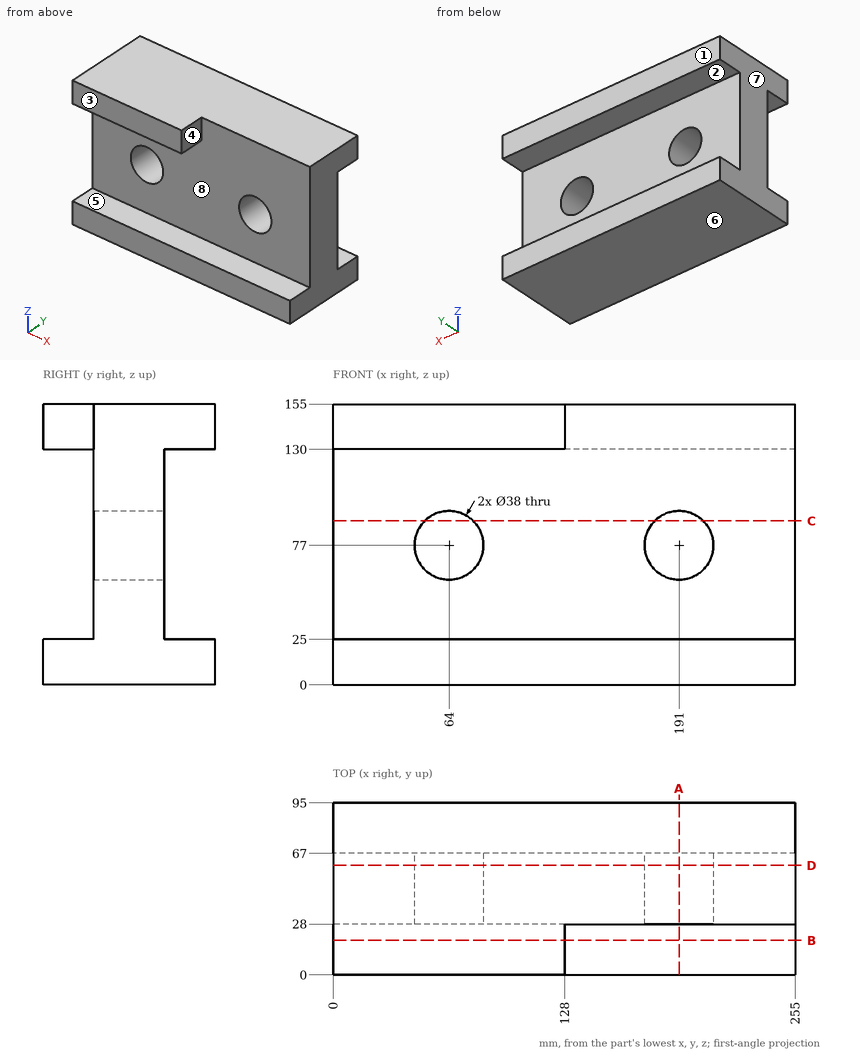
Geometry check sheet. Reference: drawing and pictorial views, mm from the part's lowest x, y, z. A direction names the side the tool comes from. Give positions to 0.01 mm unless a question says otherwise; leave off trailing zeros. Order: outer loops, then holes, each group sorted by start corner. A loop starts at its lowest first (then second) coordinate and runs counter-clockwise, first axis right, second up. Notation, with made-up numbers: M 42.5,55 L 84.5,55 A13 cw 84.5,76 Z; hole C 26,39 d5. An arc over 180 degrees is marked long. Answer as CSV lines item,"result". Start each with the question number.
Item 1: Cross-section at B-B on y = 19. Enter the section's corners in (x, z), plus the area to 4 significant figures.
Item 2: Tool access check on the marked faces 1, 2, 3, 4 and 5. Record the directions out of +Z, -Z, +X, -X, +Y, -Y that give a thin tool (end or side, any length) a straight path to the whole face; none if there is none.
Item 3: Cross-section at D-D on y = 60.5. Enter the section's corners in (x, z), plus the area to 3 significant figures.
Item 4: Gauge pin test, flat ends, axial feed: P1, Ø1.5, axis at x = 184, z = 118.5, coming from the +Y side; P2, Ø12.5, axis at y = 10.5, z = 139, coming from the +X side. Record the tip position at first contact, or that the pin passes through.
Item 5: Thickness scan on line 1 (X direction, y = 47, z = 77); line 2 (Z direction, x = 116, y = 15); line 3 (Z direction, x = 64, y = 49). Record the ranges inside material, lowest first. Write a range as [from, to].
Item 6: Mould release check, pull along Z, two halves, no side actions. Record for the marked faces 6, 7 and 8: +Z half, -Z half, draft (parallel to the pull), parting line (faces both ways), or undercut.
Item 7: Cross-section at A-A on x = 191. Enter the section's corners in (y, z).
Item 8: Cross-section at C-C on z = 90.5. Enter the section's corners in (x, y).
Established:
1,outline,"M 0,0 L 255,0 L 255,25 L 0,25 Z; M 0,130 L 128,130 L 128,155 L 0,155 Z"
1,area,"9,575 mm^2"
2,face 1,"+Z, -Z, +X, -X, +Y"
2,face 2,"+X, -X, +Y"
2,face 3,"+Z, -Z, +X, -X, -Y"
2,face 4,"+Z, +X, -Y"
2,face 5,"+X, -X, -Y"
3,outline,"M 0,0 L 255,0 L 255,155 L 0,155 Z; hole C 64,77 d38; hole C 191,77 d38"
3,area,"37,300 mm^2"
4,P1,"stops at y = 67"
4,P2,"stops at x = 128"
5,line 1,"x = [0, 45], [83, 172], [210, 255]"
5,line 2,"z = [0, 25], [130, 155]"
5,line 3,"z = [0, 58], [96, 155]"
6,face 6,"-Z half"
6,face 7,"draft"
6,face 8,"undercut"
7,outline,"M 0,0 L 95,0 L 95,25 L 67,25 L 67,58 L 28,58 L 28,25 L 0,25 Z; M 28,96 L 67,96 L 67,130 L 95,130 L 95,155 L 28,155 Z"
8,outline,"M 0,28 L 50.63,28 L 50.63,67 L 0,67 Z; M 77.37,28 L 177.63,28 L 177.63,67 L 77.37,67 Z; M 204.37,28 L 255,28 L 255,67 L 204.37,67 Z"
